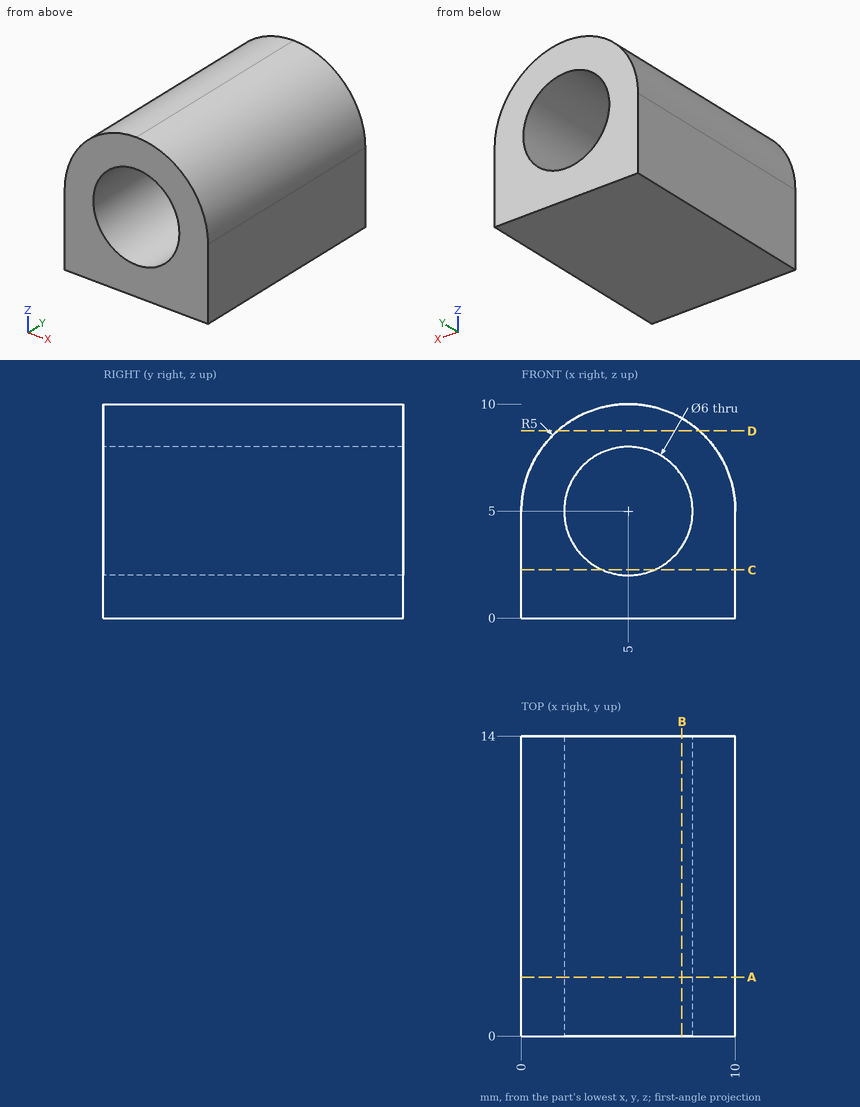
Input: dimensioned drawing with shaded views. Units: mm. Origin: part minimum x, y, z. Coordinates: 2 decimals unless noted, no trailing zeros. Write each loop counter-clockwise with the first axis right and the second up, starting at its lowest first coordinate (ties: lowest second). Pieces come first, ordered by that corner, then holes. Notation, with made-up numbers: (-25.75, 74) -> (31.25, 74) arc R7 ccw to (31.25, 78) -> close; hole circle Ø4 at (24.25, 11). An arc over 180 degrees is marked (long way). Return JSON: item names as keys, results as strings. Group by question number.
1) Ray query, line 1 along X through (y, z) = (10.25, 6.5); line 2 along Z through (x, y) = (4.25, 13.25); line 3 along Z through (x, y) = (7.5, 9). Return the intervals inside material, ascending.
2) Section query C-C, the plane z = 2.25. Return loops of the section in (x, y).
3) Contact query for a flat-ended pin moving along its axis: P1, Ø1, axis at y = 7.5, z = 8, coming from the -X side. Output: stop coordinate, or through.
4) Section query D-D, the plane z = 8.75. Return loops of the section in (x, y), plus the area to 3 significant figures.
5) Section query B-B, the plane x = 7.5. Return loops of the section in (y, z), plus the area to 3 significant figures.
6) Section query A-A, the plane y = 2.75. Return loops of the section in (x, z).
From the geometry:
{
 "1": {"line 1": "0.23 to 2.4, 7.6 to 9.77", "line 2": "0 to 2.1, 7.9 to 9.94", "line 3": "0 to 3.34, 6.66 to 9.33"},
 "2": {"outline": "(0, 0) -> (3.8, 0) -> (3.8, 14) -> (0, 14) -> close; (6.2, 0) -> (10, 0) -> (10, 14) -> (6.2, 14) -> close"},
 "3": {"P1": "x = 0.67"},
 "4": {"outline": "(1.69, 0) -> (8.31, 0) -> (8.31, 14) -> (1.69, 14) -> close", "area": "92.6 mm²"},
 "5": {"outline": "(0, 0) -> (14, 0) -> (14, 3.34) -> (0, 3.34) -> close; (0, 6.66) -> (14, 6.66) -> (14, 9.33) -> (0, 9.33) -> close", "area": "84.2 mm²"},
 "6": {"outline": "(0, 0) -> (10, 0) -> (10, 5) arc R5 ccw to (0, 5) -> close; hole circle Ø6 at (5, 5)"}
}
